For this review, take the finished solid that the model builds, in its own axes (mm). Face numbers are marked on the shaded views. A direction names the side the tool comes from. Coordinates: 2 decimals unless noted, no trailing zeros. Write each loop counter-clockwise with the first axis right and the second up, starting at its lowest first coordinate (ties: lowest second). Pieces come first, ordered by that corner, then holes.
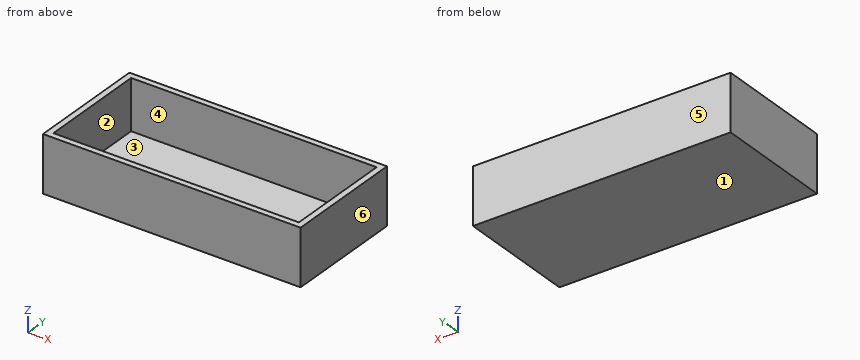
```python
from build123d import *

# Parameters (mm, degrees)
F0_W     = 812.8
F0_H     = 19.05
F1_DEPTH = 381
F2_W     = 19.05
F2_H     = 361.95
F3_DEPTH = 158.75
F5_W     = 774.7
F5_H     = 19.05
F6_DEPTH = 158.75


with BuildPart() as f1:
    # F0 (on Front) → F1 (new body)
    with BuildSketch(Plane.XZ):
        Rectangle(F0_W, F0_H)
    extrude(amount=F1_DEPTH)

    # F2 (on face) → F3 (join)
    with BuildSketch(Plane.XY.offset(9.525)):
        with Locations((-396.875, -180.975)):
            Rectangle(F2_W, F2_H)
    extrude(amount=F3_DEPTH)

    # F4: F1 across plane


with BuildPart() as f1_1:
    add(f1.part)
    add(f1.part.mirror(Plane.YZ))

    # F5 (on face) → F6 (join, through all)
    with BuildSketch(Plane.XY.offset(9.525)):
        with Locations((0, -9.525)):
            Rectangle(F5_W, F5_H)
        Polygon((387.35, -361.95), (-387.35, -361.95), (-406.4, -361.95), (-406.4, -381), (406.4, -381), (406.4, -361.95), align=None)
    extrude(amount=F6_DEPTH)


solid = f1_1.part
```
Q1. Add section B-B (y = -144). State the section outline as (x, z) points (3 decimals).
Ans:
outline: (-406.4, -9.525) - (406.4, -9.525) - (406.4, 168.275) - (387.35, 168.275) - (387.35, 9.525) - (-387.35, 9.525) - (-387.35, 168.275) - (-406.4, 168.275) - close
Q2. For probe 1 along Y at (x, z) = (-21, 132.5); probe 2 along X at (y, z) = (-290, 124); probe 3 along Z at (x, y) = (-274, -178) (3 decimals), list the stretches that pass through material, from the lowest coordinate up.
Ans:
probe 1: y = -381 to -361.95, -19.05 to 0
probe 2: x = -406.4 to -387.35, 387.35 to 406.4
probe 3: z = -9.525 to 9.525
Q3. Add section A-A (z = 116.5). State the section outline as (x, y) points.
Ans:
outline: (-406.4, -381) - (406.4, -381) - (406.4, 0) - (-406.4, 0) - close; hole (-387.35, -361.95) - (387.35, -361.95) - (387.35, -19.05) - (-387.35, -19.05) - close
Q4. Add section C-C (x = -158). State the section outline as (y, z) points (3 decimals).
Ans:
outline: (-381, -9.525) - (0, -9.525) - (0, 168.275) - (-19.05, 168.275) - (-19.05, 9.525) - (-361.95, 9.525) - (-361.95, 168.275) - (-381, 168.275) - close
Q5. Draft analysis for pull direction Y (two halves, no side actions). For the marked faces 3, 4, 5 and 6, state which applies: +Y half, -Y half, draft (parallel to the pull), parting line (faces both ways), or undercut.
Ans:
face 3: undercut
face 4: undercut
face 5: +Y half
face 6: draft
Q6. Tool access review of the marked faces 1 and 2: name each direction out of +Z, -Z, +X, -X, +Y, -Y from which nothing blocks a thin tool from reaching the whole face with its end or side.
Ans:
face 1: -Z, +X, -X, +Y, -Y
face 2: +Z
Q7. Clearance check with a flat-ended pin moving along its axis: pin 1 Ø10 at (x, y) = (-229.5, -155.5) entering from +Z (3 decimals). State where the tip first meets the part, or that it passes through.
Ans:
pin 1: stops at z = 9.525
